Verification items for the finished model (mm, model axes). Face numbers are marked on the shaded views. Give positions to 0.01 mm unless a question says otherwise; leave off trailing zeros. Loops run counter-clockwise (first coordinate to the right, second up) from the corner with the lowest first, then second, coordinate; pieces in that order, holes last. Notation, with made-up numbers: (-4, 87) - (31, 87) arc R32 ccw to (31, 118) - close; hole circle Ø7 at (-18, 41.25). An arc over 180 degrees is marked (long way). One line per question, with ' | ' between items. Start each with the question number.
1. Thickness scan on line 1 along X through (y, z) = (-2, 1.75); line 2 along X through (y, z) = (-9, 4.25); line 3 along Z through (x, y) = (-51, -1.5). Record the ranges inside material, lowest first. Write a range as from..to.
2. Section check C-C, the plane z = 15.75. Enter the section's corners in (x, y).
3. Section check A-A, the plane z = 21.5. Enter the section's corners in (x, y).
4. Section check B-B, the plane x = -73.5. Enter the section's corners in (y, z), then the cut area to 3 significant figures.
5. Mould release check, pull along Y, two halves, no side actions. Record for the marked faces 1, 2 and 3: +Y half, -Y half, draft (parallel to the pull), parting line (faces both ways), or undercut.
6. Depth check by flat-ended pin: pin 1 Ø1.5 at (y, z) = (-8, 9.5) entering from +X; pin 2 Ø5.5 at (x, y) = (-82.5, 2) entering from +Z; pin 3 Ø1.5 at (x, y) = (5, 9.5) entering from -Z. Enter the tip coordinate at first touch or a pass-through.
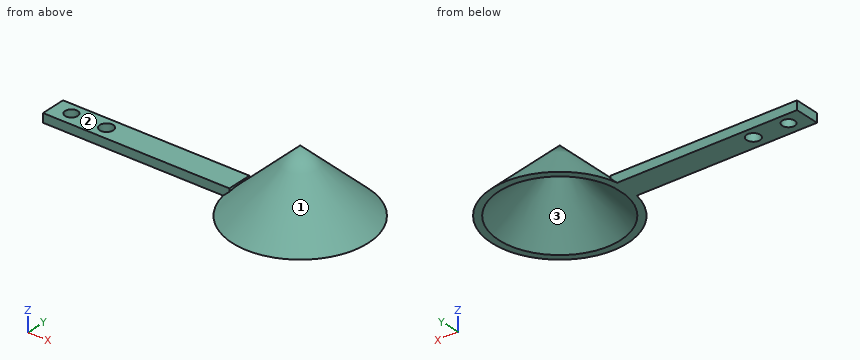
from build123d import *

# Parameters (mm, degrees)
F2_W     = 84.214361
F2_H     = 11.32601
F2_R     = 2.855499
F2_R_2   = 3.042047
F3_DEPTH = 4


with BuildPart() as f1:
    # F0 (on Front) → F1 (revolve)
    with BuildSketch(Plane.XZ):
        Polygon((0, 28.85901), (0, 26.132483), (27.431142, 0), (30.653402, 0), align=None)
    revolve(axis=Axis((0, 0, 13.066242), (0, 0, -1)))

    # F2 (on Top) → F3 (join)
    with BuildSketch(Plane.XY):
        with Locations((-69.342299, -0.36225)):
            Rectangle(F2_W, F2_H)
        with Locations((-103.411667, 0)):
            Circle(F2_R, mode=Mode.SUBTRACT)
        with Locations((-87.518722, 0)):
            Circle(F2_R_2, mode=Mode.SUBTRACT)
    extrude(amount=F3_DEPTH)


solid = f1.part
Results list:
1) line 1: -111.45..-105.45, -101.37..-89.81, -85.23..-25.52, 25.52..28.73 | line 2: -24.54..-21.13, 21.13..24.54 | line 3: 0..4
2) outline: circle Ø27.85 at (0, 0); hole circle Ø21.8 at (0, 0)
3) outline: circle Ø15.63 at (0, 0); hole circle Ø9.73 at (0, 0)
4) outline: (-6.03, 0) - (5.3, 0) - (5.3, 4) - (-6.03, 4) - close | area: 45.3 mm²
5) face 1: parting line | face 2: draft | face 3: undercut
6) pin 1: x = 19.85 | pin 2: z = 4 | pin 3: z = 15.19
